from build123d import *

# Parameters (mm, degrees)
F0_W     = 115
F0_H     = 50
F0_R     = 4.5
F1_DEPTH = 5
F2_R     = 4


with BuildPart() as f1:
    # F0 (on Top) → F1 (new body)
    with BuildSketch(Plane.XY):
        with Locations((57.5, 25)):
            Rectangle(F0_W, F0_H)
        with Locations((25.3, 25)):
            Circle(F0_R, mode=Mode.SUBTRACT)
        with Locations((89.7, 25)):
            Circle(F0_R, mode=Mode.SUBTRACT)
    extrude(amount=-F1_DEPTH)

    # F2
    f2_edges = [f1.edges().sort_by_distance(p)[0] for p in [
        (115, 0, -2.5),
        (0, 0, -2.5),
        (115, 50, -2.5),
        (0, 50, -2.5),
    ]]
    fillet(f2_edges, radius=F2_R)


solid = f1.part
Build history of the part. All positions in model axes, mm. Round coordinates to 2 decimals unless told otherwise and drop trailing zeros. Write each loop counter-clockwise with the first axis right and the second up, starting at its lowest first coordinate (ties: lowest second). Pieces come first, ordered by that corner, then holes. Notation, with made-up numbers: M 63.25,-40 L 109.25,-40 A17 ccw 109.25,-14 Z; hole C -37.75,20 d9. An arc over 180 degrees is marked long. Answer as a JSON object with one key per item and string values. Group by question number.
(1) Cut at C-C (z = -4.2). Give the cut face in (x, y).
(2) Drill centre lines: L1, parallel to Y at x = 25.3, z = -3.5; L2, parallel to X at y = 26.5, z = -3.7; L3, parallel to X at y = 24.5, z = -4.15. Where is each one in solid material? Low to high.
(3) Mould opens along Y. For faces 1 (the cylindrical face through (1.141, 1.203, -2.535)), 2 (the cylindrical face through (86.38, 28.04, -2.46)), 3 (the cylindrical face through (21.98, 28.04, -2.46)), 4 (the flat face through (0, 25, -2)) say: pulls with the +Y half, pulls with the -Y half, needs draft (parallel to the pull), parting line crosses it, or undercut.
(4) Cut at B-B (y = 25). Give the cut face in (x, z), and give its area (3 significant figures).
(5) Cut at A-A (x = 89.7). Give the cut face in (y, z), and give its area (3 significant figures).
Responses:
{
 "1": {"outline": "M 0,4 A4 ccw 4,0 L 111,0 A4 ccw 115,4 L 115,46 A4 ccw 111,50 L 4,50 A4 ccw 0,46 Z; hole C 25.3,25 d9; hole C 89.7,25 d9"},
 "2": {"L1": "y = 0 to 20.5, 29.5 to 50", "L2": "x = 0 to 21.06, 29.54 to 85.46, 93.94 to 115", "L3": "x = 0 to 20.83, 29.77 to 85.23, 94.17 to 115"},
 "3": {"face 1": "pulls with the -Y half", "face 2": "undercut", "face 3": "undercut", "face 4": "needs draft"},
 "4": {"outline": "M 0,-5 L 20.8,-5 L 20.8,0 L 0,0 Z; M 29.8,-5 L 85.2,-5 L 85.2,0 L 29.8,0 Z; M 94.2,-5 L 115,-5 L 115,0 L 94.2,0 Z", "area": "485 mm2"},
 "5": {"outline": "M 0,-5 L 20.5,-5 L 20.5,0 L 0,0 Z; M 29.5,-5 L 50,-5 L 50,0 L 29.5,0 Z", "area": "205 mm2"}
}
